Study the drawing (mm; zero at the part's minimum x, y, z) and answer. A direction names the side the tool comes from. Give positions to 0.01 mm unless a question says otherwise; leave off trailing zeros. Order: outer loops, then holes, each group sorted by start corner. A loop starts at its lowest first (then second) coordinate and runs counter-clockwise, first axis right, second up.
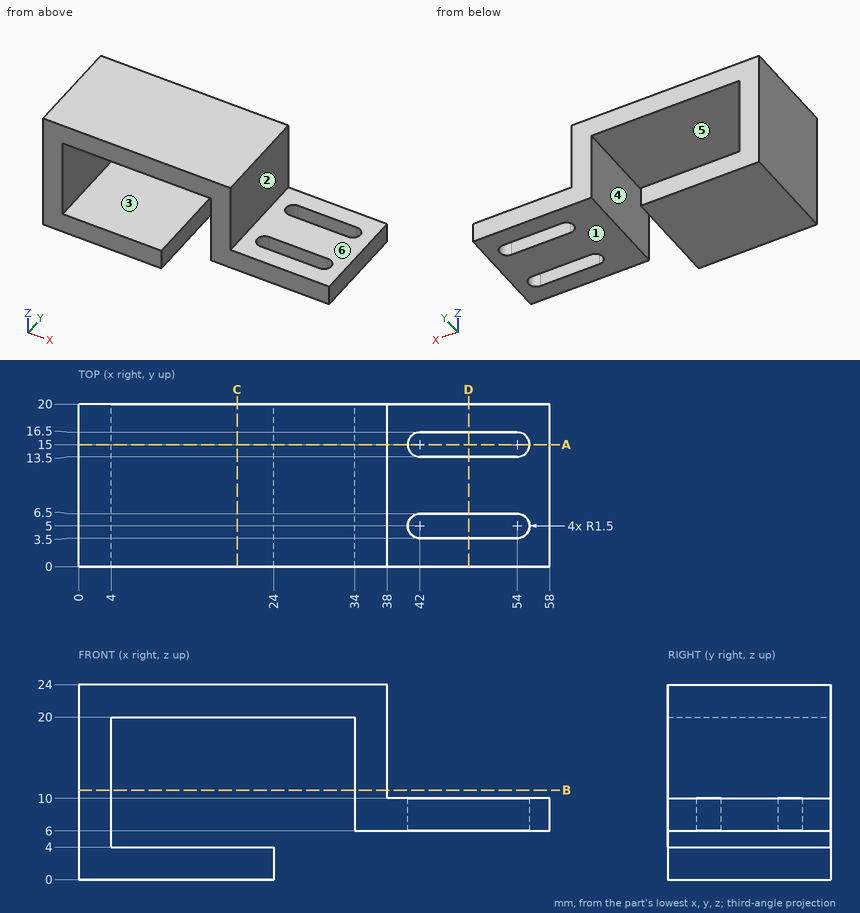
1) Find section B-B (z = 11). Write down the section's boundary in (x, y).
Geometry says:
outline: (0, 0) - (4, 0) - (4, 20) - (0, 20) - close; (34, 0) - (38, 0) - (38, 20) - (34, 20) - close
2) Given P1, Ø1.5, axis at x = 38, y = 11, coming from the -Z side; P2, Ø5, axis at x = 50, y = 15.5, coming from the +Z side; P3, Ø2, axis at y = 5.5, z = 20, coming from the +X side; P4, Ø2, axis at x = 20.5, z = 6, coming from the -Y side (3 decimals), each flat-ended and moving along its own axis, determine where each tip first touches the part or whether it passes through.
Geometry says:
P1: stops at z = 6
P2: stops at z = 10
P3: stops at x = 38
P4: passes through
3) A tool of negligible diameter and unlimited length cuts with its end or side. For the marked faces 4, 5 and 6, from which of +Z, -Z, +X, -X, +Y, -Y can it reach the whole face along a straight path? Write none if from no direction.
Geometry says:
face 4: -Z, +Y, -Y
face 5: +Y, -Y
face 6: +Z, +X, +Y, -Y
4) Find section C-C (x = 19.5). Write down the section's boundary in (y, z).
Geometry says:
outline: (0, 0) - (20, 0) - (20, 4) - (0, 4) - close; (0, 20) - (20, 20) - (20, 24) - (0, 24) - close
5) Find section A-A (y = 15). Write down the section's boundary in (x, z), then the cut area to 3 significant figures.
Geometry says:
outline: (0, 0) - (24, 0) - (24, 4) - (4, 4) - (4, 20) - (34, 20) - (34, 6) - (40.5, 6) - (40.5, 10) - (38, 10) - (38, 24) - (0, 24) - close; (55.5, 6) - (58, 6) - (58, 10) - (55.5, 10) - close
area: 388 mm2
6) Find section D-D (x = 48). Write down the section's boundary in (y, z).
Geometry says:
outline: (0, 6) - (3.5, 6) - (3.5, 10) - (0, 10) - close; (6.5, 6) - (13.5, 6) - (13.5, 10) - (6.5, 10) - close; (16.5, 6) - (20, 6) - (20, 10) - (16.5, 10) - close
7) For a pull along Z with two mould halves and no side action, classify the marked faces 1, 2 and 3 as +Z half, -Z half, draft (parallel to the pull), parting line (faces both ways), or undercut.
Geometry says:
face 1: -Z half
face 2: draft
face 3: undercut
8) Straight lines are drawn through the part: probe 1 along Y at (x, z) = (50, 8.25); probe 2 along X at (y, z) = (10.75, 15.25); probe 3 along Z at (x, y) = (12, 19). For each, find the intervals that lie inside material, in ascending order.
Geometry says:
probe 1: y = 0 to 3.5, 6.5 to 13.5, 16.5 to 20
probe 2: x = 0 to 4, 34 to 38
probe 3: z = 0 to 4, 20 to 24
